Part print with two shaded views. Sizes in mm from the minimum x, y, z corner. A direction names the side the tool comes from. Round coordinates to 2 decimals unless told otherwise and drop trailing zeros. Order: outer loops, then holes, each group sorted by start corner. A loop starts at its lowest first (then second) coordinate and runs counter-clockwise, first axis right, second up. Notation, with made-up numbers: (-37.75, 60.5) -> (-12.75, 60.5) arc R31 ccw to (-12.75, 98.5) -> close; hole circle Ø9 at (-21, 1). An arc over 180 degrees is marked (long way). Answer as a JSON object with one key per item and string values.
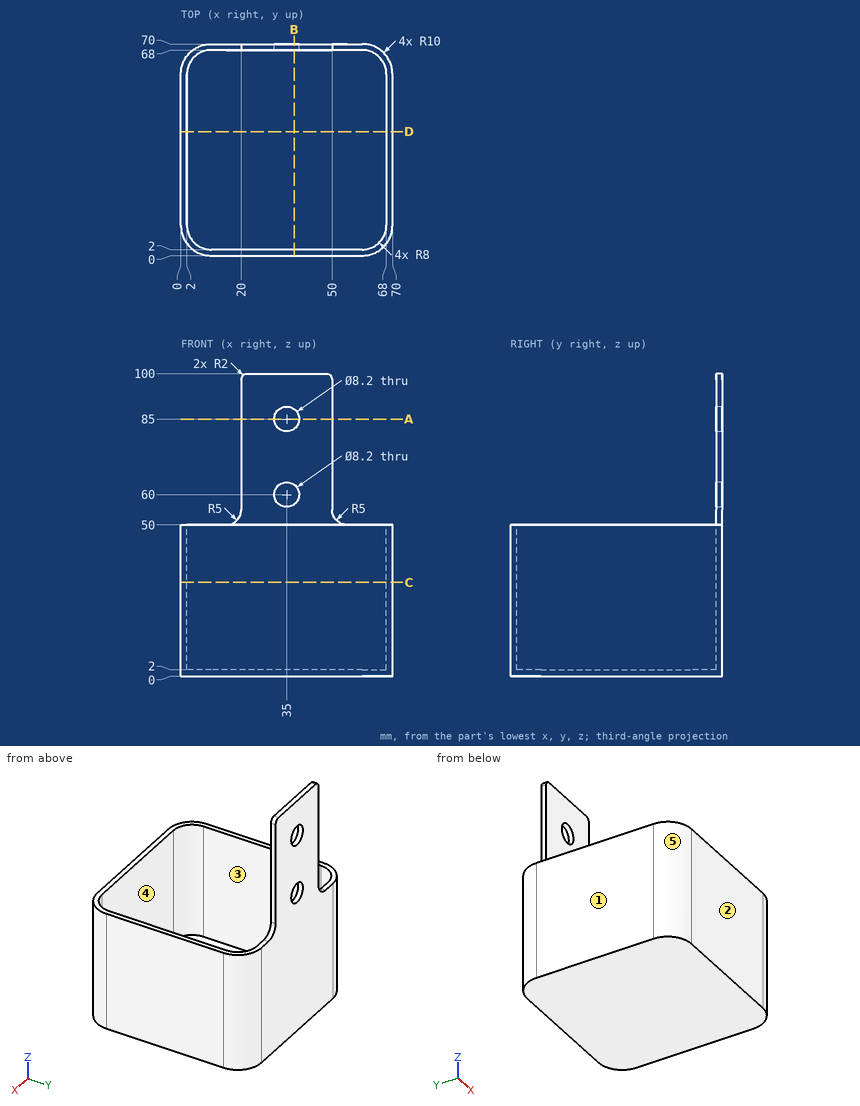
1) Which spindle directions (+Z, -Z, +X, -X, +Y, -Y) get a long thin tool onto all of the face, cutting with end or side? Do the marked faces 4 and 5. Say none if no direction does.
Checked values:
{"face 4": "+Z", "face 5": "+Z, -Z, -X, -Y"}
2) Cut at C-C, the plane z = 31. Give the cut face in (x, y), plus the area to 3 significant figures.
Checked values:
{"outline": "(0, 10) arc R10 ccw to (10, 0) -> (60, 0) arc R10 ccw to (70, 10) -> (70, 60) arc R10 ccw to (60, 70) -> (10, 70) arc R10 ccw to (0, 60) -> close; hole (2, 10) arc R8 ccw to (10, 2) -> (60, 2) arc R8 ccw to (68, 10) -> (68, 60) arc R8 ccw to (60, 68) -> (10, 68) arc R8 ccw to (2, 60) -> close", "area": "513 mm²"}
3) Pull direction X, two halves, no side cores. Call the marked faces 1, 2 and 3: pulls with the +X half, pulls with the -X half, needs draft (parallel to the pull), parting line crosses it, or undercut.
Checked values:
{"face 1": "pulls with the -X half", "face 2": "needs draft", "face 3": "undercut"}
4) Cut at D-D, the plane y = 41. Give the cut face in (x, z).
Checked values:
{"outline": "(0, 0) -> (70, 0) -> (70, 50) -> (68, 50) -> (68, 2) -> (2, 2) -> (2, 50) -> (0, 50) -> close"}
5) Probe L1, parallel to Y at x = 20.5, z = 47; L2, parallel to X at y = 68.6, z = 60. List the from-to ranges inside material, lowest first. Write a range as from..to.
Checked values:
{"L1": "y = 0..2, 68..70", "L2": "x = 20..30.9, 39.1..50"}
6) Cut at B-B, the plane x = 37.5. Give the cut face in (y, z), plus the area to 3 significant figures.
Checked values:
{"outline": "(0, 0) -> (70, 0) -> (70, 56.75) -> (68, 56.75) -> (68, 2) -> (2, 2) -> (2, 50) -> (0, 50) -> close; (68, 63.25) -> (70, 63.25) -> (70, 81.75) -> (68, 81.75) -> close; (68, 88.25) -> (70, 88.25) -> (70, 100) -> (68, 100) -> close", "area": "406 mm²"}
7) Cut at A-A, the plane z = 85. Give the cut face in (x, y), plus the area to 3 significant figures.
Checked values:
{"outline": "(20, 68) -> (30.9, 68) -> (30.9, 70) -> (20, 70) -> close; (39.1, 68) -> (50, 68) -> (50, 70) -> (39.1, 70) -> close", "area": "43.6 mm²"}
8) Flat gauge pins, fed straight in: pin 1 Ø2 at (y, z) = (68.5, 75) entering from -X; pin 2 Ø1 at (y, z) = (69, 68) entering from +X; pin 3 Ø21 at (x, y) = (51.5, 31) entering from +Z. Where does each tip first touch, or does it go through?
Checked values:
{"pin 1": "stops at x = 20", "pin 2": "stops at x = 50", "pin 3": "stops at z = 2"}
